The listing builds one solid part. Answer for the finished solid, in the listing's coordinates (mm). Face numbers are marked on the shaded views. A direction names the side the tool comes from. Give positions to 0.01 mm unless a question says otherwise; leave off trailing zeros. Order: outer loops, then holes, each group sorted by start corner. A loop starts at its lowest first (then second) coordinate and runs counter-clockwise, first axis right, second up. Notation, with made-up numbers: (-1.75, 84) -> (26.25, 84) arc R38 cw to (26.25, 122) -> close; hole circle Ø6 at (-1, -21). An arc over 180 degrees is marked (long way). Answer as a JSON object with one key per item and string values. Group by question number.
```python
from build123d import *

# Parameters (mm, degrees)
ESQUISSE2_R      = 1.5
EXTRUSION1_DEPTH = 10
ESQUISSE3_R      = 2.75
EXTRUSION2_DEPTH = 3
CHANFREIN1_SIZE  = 0.5


with BuildPart() as part:
    # Esquisse2 → Extrusion1 (new body)
    with BuildSketch(Plane.XY):
        Circle(ESQUISSE2_R)
    extrude(amount=EXTRUSION1_DEPTH)

    # Esquisse3 → Extrusion2 (add)
    with BuildSketch(Plane(origin=(0, 0, 0), x_dir=(-1, 0, 0), z_dir=(0, 0, -1))):
        Circle(ESQUISSE3_R)
    extrude(amount=EXTRUSION2_DEPTH)

    # Chanfrein1
    chanfrein1_edges = [part.edges().sort_by_distance(p)[0] for p in [
        (-1.5, 0, 10),
    ]]
    chamfer(chanfrein1_edges, length=CHANFREIN1_SIZE)


solid = part.part
```
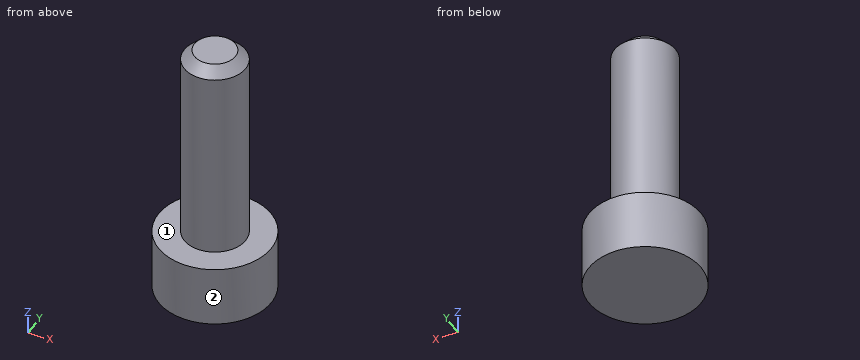
(1) Find the intervals of material crossed by line 1 along Z through (x, y) = (-1.1, -2.05); line 2 along Y through (x, z) = (0.05, 6.5); line 3 along X through (y, z) = (0.85, -0.25), in increasing order. Write a range as [from, to].
(2) Which of the six approach directions +Z, -Z, +X, -X, +Y, -Y give full straight-line access (tool end or side, diameter ignored) to the marked faces 1 and 2?
(3) A cutting plane is placed at C-C (z = 2). Determine the outline of the cut face in (x, y), and give its area (3 significant figures).
(4) A cutting plane is placed at A-A (x = 0). Determine the outline of the cut face in (y, z), and give its area (4 significant figures).
(5) A cutting plane is placed at D-D (x = 2.1). Determine the outline of the cut face in (y, z).
(6) Flat-ended cylindrical pins translate along their axes: pin 1 Ø2 at (x, z) = (1.5, 2) entering from +Y; pin 2 Ø2 at (y, z) = (-1.5, 4) entering from -X; pin 3 Ø3 at (x, z) = (1, 7.5) entering from -Y. Find the tip coordinate at first contact, or state that the pin passes through.
Check sheet entries:
{
 "1": {"line 1": "z = [-3, 0]", "line 2": "y = [-1.5, 1.5]", "line 3": "x = [-2.62, 2.62]"},
 "2": {"face 1": "+Z", "face 2": "+Z, -Z"},
 "3": {"outline": "circle Ø3 at (0, 0)", "area": "7.07 mm2"},
 "4": {"outline": "(-2.75, -3) -> (2.75, -3) -> (2.75, 0) -> (1.5, 0) -> (1.5, 9.5) -> (1, 10) -> (-1, 10) -> (-1.5, 9.5) -> (-1.5, 0) -> (-2.75, 0) -> close", "area": "46.25 mm2"},
 "5": {"outline": "(-1.78, -3) -> (1.78, -3) -> (1.78, 0) -> (-1.78, 0) -> close"},
 "6": {"pin 1": "stops at y = 1.41", "pin 2": "stops at x = -1.41", "pin 3": "stops at y = -1.5"}
}
